The drawing under review shows one solid part. Ordinate dimensions are in mm from its lowest x, y, z. Coordinates: 2 decimals unless noted, no trailing zeros. Loops run counter-clockwise (first coordinate to the right, second up) from the corner with the lowest first, then second, coordinate; pieces in that order, holes last. Notation, with made-up numbers: M 3,62 L 43,62 A12 ccw 43,81 Z; hole C 38.5,2.25 d3. An arc over 180 degrees is marked long. Use one line per item in the form item = value.
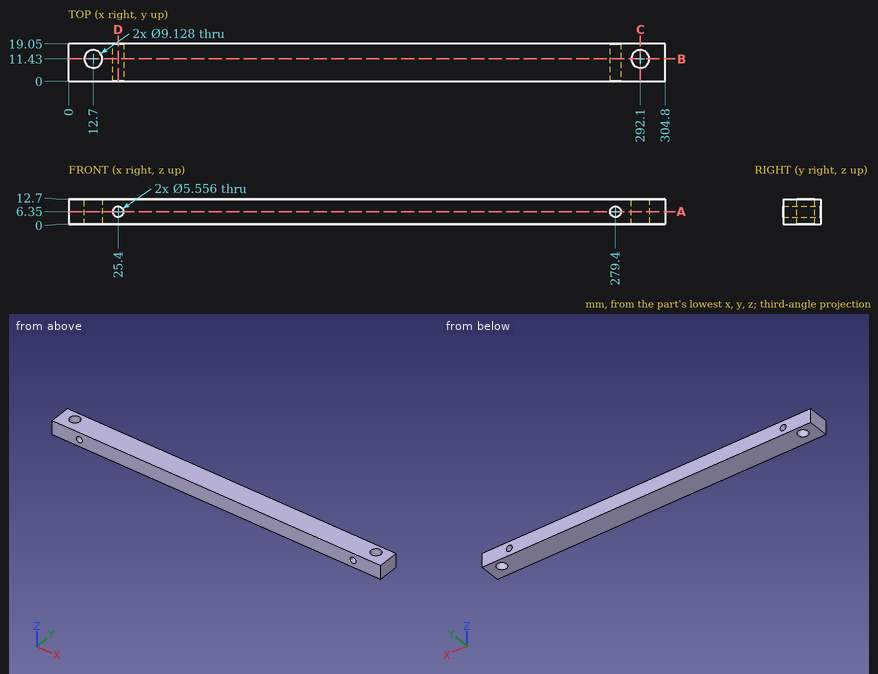
1. Consider section C-C on x = 292.1. Write out the cut boundary in (y, z).
Computed values:
outline = M 0,0 L 6.87,0 L 6.87,12.7 L 0,12.7 Z; M 15.99,0 L 19.05,0 L 19.05,12.7 L 15.99,12.7 Z
2. Consider section B-B on y = 11.43. Write out the cut boundary in (x, z).
Computed values:
outline = M 0,0 L 8.14,0 L 8.14,12.7 L 0,12.7 Z; M 17.26,0 L 287.54,0 L 287.54,12.7 L 17.26,12.7 Z; M 296.66,0 L 304.8,0 L 304.8,12.7 L 296.66,12.7 Z; hole C 25.4,6.35 d5.56; hole C 279.4,6.35 d5.56
3. Wall thickness on line 1 along Z through (x, y) = (25.4, 5.25); line 2 along X through (y, z) = (7.75, 6.35); line 3 along X through (y, z) = (12.5, 3.25): over which ranges is each line inside the solid? List them lowest first. Write a range as from..to.
Computed values:
line_1 = 0..3.57, 9.13..12.7
line_2 = 0..10, 15.4..22.62, 28.18..276.62, 282.18..289.4, 294.8..304.8
line_3 = 0..8.26, 17.14..287.66, 296.54..304.8
4. Consider section D-D on x = 25.4. Write out the cut boundary in (y, z).
Computed values:
outline = M 0,0 L 19.05,0 L 19.05,3.57 L 0,3.57 Z; M 0,9.13 L 19.05,9.13 L 19.05,12.7 L 0,12.7 Z
5. Consider section A-A on z = 6.35. Write out the cut boundary in (x, y).
Computed values:
outline = M 0,0 L 22.62,0 L 22.62,19.05 L 0,19.05 Z; M 28.18,0 L 276.62,0 L 276.62,19.05 L 28.18,19.05 Z; M 282.18,0 L 304.8,0 L 304.8,19.05 L 282.18,19.05 Z; hole C 12.7,11.43 d9.13; hole C 292.1,11.43 d9.13
